from build123d import *

# Parameters (mm, degrees)
F0_W     = 65
F0_H     = 93.7
F1_DEPTH = 30
F2_W     = 65
F2_H     = 14.8
F3_DEPTH = 11.7
F4_W     = 65
F4_H     = 5.2
F5_DEPTH = 11.7
F6_W     = 50
F6_H     = 40
F7_DEPTH = 25


with BuildPart() as f1:
    # F0 (on Top) → F1 (new body)
    with BuildSketch(Plane.XY):
        Rectangle(F0_W, F0_H)
    extrude(amount=F1_DEPTH)

    # F2 (on face) → F3 (cut)
    with BuildSketch(Plane(origin=(0, 46.85, 0), x_dir=(-1, 0, 0), z_dir=(0, 1, 0))):
        with Locations((0, 22.6)):
            Rectangle(F2_W, F2_H)
    extrude(amount=-F3_DEPTH, mode=Mode.SUBTRACT)

    # F4 (on face) → F5 (cut)
    with BuildSketch(Plane(origin=(0, 46.85, 0), x_dir=(-1, 0, 0), z_dir=(0, 1, 0))):
        with Locations((0, 2.6)):
            Rectangle(F4_W, F4_H)
    extrude(amount=-F5_DEPTH, mode=Mode.SUBTRACT)

    # F6 (on face) → F7 (cut)
    with BuildSketch(Plane.XY.offset(30)):
        with Locations((0, -16.85)):
            Rectangle(F6_W, F6_H)
    extrude(amount=-F7_DEPTH, mode=Mode.SUBTRACT)


solid = f1.part
Can you work these out from the model? Positions are in its coordinate system, mm. A direction names the side the tool comes from. Round coordinates to 2 decimals unless told otherwise and drop trailing zeros. Loops run counter-clockwise (first coordinate to the right, second up) from the corner with the lowest first, then second, coordinate; pieces in that order, holes last. Notation, with made-up numbers: (-29.75, 26.25) - (29.25, 26.25) arc R20 ccw to (29.25, 40.25) - close; hole circle Ø10 at (37.25, -22.75). An arc over 180 degrees is marked (long way). Answer in a Markdown table with one row per item. Add a question column.
Q1. For pin 1 Ø12 at (x, z) = (1, 24) entering from +Y; pin 2 Ø9.5 at (x, y) = (-9.5, 43) entering from -Z, each with a flat end and sliding along its axis, tell me the tip position at first contact or that it passes through.
Q2. Which directions (+Z, -Z, +X, -X, +Y, -Y) give clear straight access to the entire face, cutting with the end or side of a thin tool? Please do faces 1 (the flat face through (0, -36.85, 18)), 2 (the flat face through (0, 35.15, 23)), 3 (the flat face through (0, 35.15, 3)), 4 (the flat face through (0, -46.85, 15)), 5 (the flat face through (0, 4, 30)).
Q3. I need wall thicknesses on L1, parallel to X at y = -30, z = 10.5; L2, parallel to Y at x = -15.5, z = 25.75; L3, parallel to Y at x = -22, z = 8.5. Which ranges of each line are inside material? Lowest first, please.
Q4. I want a section at C-C on y = -29. List the corners of the cut face in (x, z) for me, and give its area (3 significant figures).
Q5. I want a section at A-A on z = 7.5. List the corners of the cut face in (x, y) for me.
Q6. I want a section at D-D on z = 23.5. List the corners of the cut face in (x, y) for me.
Q7. I want a section at B-B on x = 4.5. List the corners of the cut face in (y, z) for me, and give its area (3 significant figures).
A:
| question | item | result |
|---|---|---|
| 1 | pin 1 | y = 35.15 |
| 1 | pin 2 | z = 5.2 |
| 2 | face 1 | +Z |
| 2 | face 2 | +Z, +X, -X, +Y |
| 2 | face 3 | -Z, +X, -X, +Y |
| 2 | face 4 | +Z, -Z, +X, -X, -Y |
| 2 | face 5 | +Z, +X, -X, +Y, -Y |
| 3 | L1 | -32.5 to -25, 25 to 32.5 |
| 3 | L2 | -46.85 to -36.85, 3.15 to 35.15 |
| 3 | L3 | -46.85 to -36.85, 3.15 to 46.85 |
| 4 | outline | (-32.5, 0) - (32.5, 0) - (32.5, 30) - (25, 30) - (25, 5) - (-25, 5) - (-25, 30) - (-32.5, 30) - close |
| 4 | area | 700 mm^2 |
| 5 | outline | (-32.5, -46.85) - (32.5, -46.85) - (32.5, 46.85) - (-32.5, 46.85) - close; hole (-25, -36.85) - (25, -36.85) - (25, 3.15) - (-25, 3.15) - close |
| 6 | outline | (-32.5, -46.85) - (32.5, -46.85) - (32.5, 35.15) - (-32.5, 35.15) - close; hole (-25, -36.85) - (25, -36.85) - (25, 3.15) - (-25, 3.15) - close |
| 7 | outline | (-46.85, 0) - (35.15, 0) - (35.15, 5.2) - (46.85, 5.2) - (46.85, 15.2) - (35.15, 15.2) - (35.15, 30) - (3.15, 30) - (3.15, 5) - (-36.85, 5) - (-36.85, 30) - (-46.85, 30) - close |
| 7 | area | 1,580 mm^2 |
